Check sheet for the modelled part. Datum: model origin and axes. Units: mm. A direction names the side the tool comes from. Round coordinates to 2 decimals unless told otherwise and drop trailing zeros. Write each loop counter-clockwise with the first axis right and the second up, starting at its lowest first coordinate (ties: lowest second). Pieces come first, ordered by that corner, then holes.
Item 1: Cross-section at A-A on x = -5. Enter the section's corners in (y, z).
Item 2: Cross-section at B-B on z = 563.5. Enter the section's corners in (x, y), plus the area to 3 significant figures.
Item 3: Material ranges on line 1 (Y direction, x = -8, z = 269.5); line 2 (X direction, y = -15, z = 379), recorded low to high.
Item 4: Tool access check on faces 1 (the flat face through (-15.9, 0, 339)), 2 (the flat face through (17.5, 0, 339)). Record the directions out of +Z, -Z, +X, -X, +Y, -Y that give a thin tool (end or side, any length) a straight path to the whole face; none if there is none.
Item 5: Release check for a two-part mould opening along X. For faces 3 (the flat face through (0, -17, 688)), 4 (the flat face through (15.9, 0, 339)), 5 (the flat face through (0, -17.5, 339)) record: +X half, -X half, draft (parallel to the pull), parting line (faces both ways), or undercut.
Item 6: Cross-section at C-C on y = -2.5. Enter the section's corners in (x, z), plus the area to 3 significant figures.
Autodesk Inventor part; units mm, degrees
ref_plane "Start plane" through (0, 0, -17.5) normal (0, 0, 1) x (1, 0, 0)
ref_plane "End plane" through (0, 0, 705.5) normal (0, 0, 1) x (1, 0, 0)
ref_plane "Work Plane20" through (-20.2643, 0, 0.3072) normal (-0.871, 0, -0.4912) x (-0.4912, 0, 0.871)
ref_plane "Start plane" through (0, 0, -17.5) normal (0, 0, 1) x (1, 0, 0)
ref_plane "End plane" through (0, 0, 705.5) normal (0, 0, 1) x (1, 0, 0)
sketch "Sketch" plane through (0, 0, 0) normal (0, 0, 1) x (1, 0, 0)
  line L0 (-17.5, -14.3) -> (-17.5, 14.3)
  line L1 (-14.3, 17.5) -> (14.3, 17.5)
  line L2 (17.5, 14.3) -> (17.5, -14.3)
  line L3 (14.3, -17.5) -> (-14.3, -17.5)
  arc A0 (-17.5, -14.3) -> (-14.3, -17.5) centre (-14.3, -14.3) ccw
  arc A1 (-14.3, 17.5) -> (-17.5, 14.3) centre (-14.3, 14.3) ccw
  arc A2 (17.5, 14.3) -> (14.3, 17.5) centre (14.3, 14.3) ccw
  arc A3 (14.3, -17.5) -> (17.5, -14.3) centre (14.3, -14.3) ccw
  arc A4 (-14.3, 15.9) -> (-15.9, 14.3) centre (-14.3, 14.3) ccw
  line L4 (-14.3, 15.9) -> (14.3, 15.9)
  arc A5 (15.9, 14.3) -> (14.3, 15.9) centre (14.3, 14.3) ccw
  line L5 (15.9, 14.3) -> (15.9, -14.3)
  arc A6 (14.3, -15.9) -> (15.9, -14.3) centre (14.3, -14.3) ccw
  line L6 (14.3, -15.9) -> (-14.3, -15.9)
  arc A7 (-15.9, -14.3) -> (-14.3, -15.9) centre (-14.3, -14.3) ccw
  line L7 (-15.9, -14.3) -> (-15.9, 14.3)
  line L8 (0, 25.4278) -> (0, -25.4278) construction
  line L9 (-25.4278, 0) -> (25.4278, 0) construction
  dimension "d7" = 3.2
  dimension "d10" = 35
  dimension "d11" = 35
  dimension "d12" = 1.6
  dimension "d15" = 17.5
  dimension "d16" = 17.5
extrude "Body" add sketch "Sketch" along normal up to surface (723 mm away) from surface at -17.5
sketch "Sketch3" plane through (0, 0, 0) normal (0, 0, 1) x (1, 0, 0)
  line L0 (0, 0) -> (10, 0)
ref_plane "Work Plane3" through (0, 0, 0) normal (0, -1, 0) x (1, 0, 0)
sketch "Sketch4" plane through (0, 0, 0) normal (0, -1, 0) x (1, 0, 0)
  line L0 (-2, -17.5) -> (12, -17.5)
  line L1 (-2, 705.5) -> (12, 705.5)
  dimension "d18" = 723
ref_plane "Work Plane20" through (-20.2643, 0, 0.3072) normal (-0.871, 0, -0.4912) x (-0.4912, 0, 0.871)
split "Split5" plane through (-20.2643, 0, 0.3072) removes the side toward (-0.871, 0, -0.4912)
ref_plane "Work Plane21" through (-20.2643, 0, 687.6928) normal (-0.871, 0, 0.4912) x (0.4912, 0, 0.871)
split "Split6" plane through (-20.2643, 0, 687.6928) removes the side toward (-0.871, 0, 0.4912)
ref_plane "Work Plane22" through (17.5, 0, 705.5) normal (-0.7071, 0, 0.7071) x (0.7071, 0, 0.7071)
split "Split7" plane through (17.5, 0, 705.5) removes the side toward (-0.7071, 0, 0.7071)
ref_plane "Work Plane23" through (17.5, 0, -17.5) normal (-0.7071, 0, -0.7071) x (-0.7071, 0, 0.7071)
split "Split8" plane through (17.5, 0, -17.5) removes the side toward (-0.7071, 0, -0.7071)
equation "\"d7\" = G_IR"
equation "\"d10\" = G_H"
equation "\"d11\" = G_W"
equation "\"d12\" = G_T"
equation "\"d15\" = 0.5 * d10"
equation "\"d16\" = 0.5 * d11"
equation "\"d3\" = G_L"
equation "\"G_W\" = 35"
equation "\"G_H\" = 35"
equation "\"G_T\" = 1.6"
equation "\"G_IR\" = 3.2"
equation "\"G_L\" = d18"
equation "\"G_OFFSET_START\" = 17.5"
equation "\"G_OFFSET_END\" = 17.5"
equation "\"d13\" = -G_OFFSET_START"
equation "\"d14\" = G_OFFSET_END + B_L"
equation "\"B_L\" = 688"
properties part number "AS 1163 - C350L0 35x35x1.6 SHS - 723" material "Steel, Mild"
Response values:
1. outline: (-17.5, 5) - (-15.9, 5) - (-15.9, 683) - (-17.5, 683) - close; (15.9, 5) - (17.5, 5) - (17.5, 683) - (15.9, 683) - close
2. outline: (-17.5, -14.3) arc R3.2 ccw to (-14.3, -17.5) - (14.3, -17.5) arc R3.2 ccw to (17.5, -14.3) - (17.5, 14.3) arc R3.2 ccw to (14.3, 17.5) - (-14.3, 17.5) arc R3.2 ccw to (-17.5, 14.3) - close; hole (-15.9, -14.3) arc R1.6 ccw to (-14.3, -15.9) - (14.3, -15.9) arc R1.6 ccw to (15.9, -14.3) - (15.9, 14.3) arc R1.6 ccw to (14.3, 15.9) - (-14.3, 15.9) arc R1.6 ccw to (-15.9, 14.3) - close
2. area: 207 mm2
3. line 1: y = -17.5 to -15.9, 15.9 to 17.5
3. line 2: x = -17.42 to -15.74, 15.74 to 17.42
4. face 1: +Z, -Z
4. face 2: +Z, -Z, +X, +Y, -Y
5. face 3: -X half
5. face 4: undercut
5. face 5: draft
6. outline: (-17.5, 17.5) - (-15.9, 15.9) - (-15.9, 672.1) - (-17.5, 670.5) - close; (15.9, -15.9) - (17.5, -17.5) - (17.5, 705.5) - (15.9, 703.9) - close
6. area: 2,200 mm2
